Build history of the part. All positions in model axes, mm. A direction names the side the tool comes from. Coordinates: 2 decimals unless noted, no trailing zeros. Loops run counter-clockwise (first coordinate to the right, second up) from the corner with the lowest first, then second, coordinate; pieces in that order, holes last.
(1) Slice it at A-A (y = 4.5). Give the cut face in (x, z), and give its area (3 significant figures).
(2) Two-plate mould, pull along X, no slides. Class faces 1 (the face through (0, -11, 7)), 2 (the face through (-13.887, -10.648, 13.395)): pulls with the +X half, pulls with the -X half, needs draft (parallel to the pull), parting line crosses it, or undercut.
(3) Slice it at D-D (x = -7). Give the cut face in (y, z), and give its area (3 significant figures).
(4) Slice it at B-B (x = 24.5). Give the cut face in (y, z), and give its area (3 significant figures).
(5) Tool access for faces 3 (the face through (9.54, -7.32, 3.45)), 4 (the face through (-29.97, 1.32, 2.46)), 5 (the face through (7.94, 13.6, 16.07)): list every direction of +Z, -Z, +X, -X, +Y, -Y with a clear straight run to the whole face (end or side of a thin tool).
(6) Flat gauge pins, fed straight in: P1, Ø6, axis at x = -3, z = 11, coming from the -Y side; P2, Ø2, axis at x = -4.5, z = 9.5, coming from the +Y side; P3, Ø4, axis at y = -0.5, z = 10.5, coming from the +X side. Where does each tip first touch, or does it go through?
(7) Wall check: L1, parallel to Y at x = 12.25, z = 1.6; L2, parallel to X at y = -13.5, z = 11.75; L3, parallel to Y at x = -11, z = 2.25. Give the ranges that are in metal, low to high.
(8) Slice it at C-C (z = 8.25). Give the cut face in (x, y), and give its area (3 significant figures).
from build123d import *

# Parameters (mm, degrees)
SKETCH1_R           = 30
BOSS_EXTRUDE1_DEPTH = 5
SKETCH2_R           = 19.5
BOSS_EXTRUDE2_DEPTH = 1
SKETCH3_R           = 17.5
BOSS_EXTRUDE3_DEPTH = 15
SKETCH4_R           = 12.025
CUT_EXTRUDE1_DEPTH  = 7
SKETCH5_R           = 10.5
CUT_EXTRUDE2_DEPTH  = 45.676615807
SKETCH6_R           = 1.75
CUT_EXTRUDE3_DEPTH  = 46.343136195
SKETCH7_R           = 1.75
CUT_EXTRUDE4_DEPTH  = 10
SKETCH8_R           = 1.225
CUT_EXTRUDE5_DEPTH  = 12


with BuildPart() as part:
    # Sketch1 → Boss-Extrude1 (new body)
    with BuildSketch(Plane.XY):
        Circle(SKETCH1_R)
    extrude(amount=BOSS_EXTRUDE1_DEPTH)

    # Sketch2 → Boss-Extrude2 (add)
    with BuildSketch(Plane.XY.offset(5)):
        Circle(SKETCH2_R)
    extrude(amount=BOSS_EXTRUDE2_DEPTH)

    # Sketch3 → Boss-Extrude3 (add)
    with BuildSketch(Plane.XY.offset(6)):
        Circle(SKETCH3_R)
    extrude(amount=BOSS_EXTRUDE3_DEPTH)

    # Sketch4 → Cut-Extrude1 (cut)
    with BuildSketch(Plane(origin=(0, 0, 0), x_dir=(-1, 0, 0), z_dir=(0, 0, -1))):
        Circle(SKETCH4_R)
    extrude(amount=-CUT_EXTRUDE1_DEPTH, mode=Mode.SUBTRACT)

    # Sketch5 → Cut-Extrude2 (cut, through all)
    with BuildSketch(Plane(origin=(0, 0, 7), x_dir=(-1, 0, 0), z_dir=(0, 0, -1))):
        Circle(SKETCH5_R)
    extrude(amount=-CUT_EXTRUDE2_DEPTH, mode=Mode.SUBTRACT)

    # Sketch6 → Cut-Extrude3 (cut, through all)
    with BuildSketch(Plane.XY.offset(5)):
        with Locations((24.5, 0)):
            Circle(SKETCH6_R)
        with Locations((12.25, -21.217622393)):
            Circle(SKETCH6_R)
        with Locations((-12.25, -21.217622393)):
            Circle(SKETCH6_R)
        with Locations((-24.5, 0)):
            Circle(SKETCH6_R)
        with Locations((-12.25, 21.217622393)):
            Circle(SKETCH6_R)
        with Locations((12.25, 21.217622393)):
            Circle(SKETCH6_R)
    extrude(amount=-CUT_EXTRUDE3_DEPTH, mode=Mode.SUBTRACT)

    # Sketch7 → Cut-Extrude4 (cut)
    with BuildSketch(Plane.XY.offset(21)):
        with Locations((14, 0)):
            Circle(SKETCH7_R)
        with Locations((7, -12.124355653)):
            Circle(SKETCH7_R)
        with Locations((-7, -12.124355653)):
            Circle(SKETCH7_R)
        with Locations((-14, 0)):
            Circle(SKETCH7_R)
        with Locations((-7, 12.124355653)):
            Circle(SKETCH7_R)
        with Locations((7, 12.124355653)):
            Circle(SKETCH7_R)
    extrude(amount=-CUT_EXTRUDE4_DEPTH, mode=Mode.SUBTRACT)

    # Sketch8 → Cut-Extrude5 (cut)
    with BuildSketch(Plane.XY.offset(21)):
        with Locations((12.124355653, 7)):
            Circle(SKETCH8_R)
        with Locations((0, -14)):
            Circle(SKETCH8_R)
        with Locations((-12.124355653, 7)):
            Circle(SKETCH8_R)
    extrude(amount=-CUT_EXTRUDE5_DEPTH, mode=Mode.SUBTRACT)


solid = part.part
Response values:
1. outline: (-29.66, 0) - (-11.15, 0) - (-11.15, 7) - (-9.49, 7) - (-9.49, 21) - (-16.91, 21) - (-16.91, 6) - (-18.97, 6) - (-18.97, 5) - (-29.66, 5) - close; (9.49, 7) - (11.15, 7) - (11.15, 0) - (29.66, 0) - (29.66, 5) - (18.97, 5) - (18.97, 6) - (16.91, 6) - (16.91, 21) - (9.49, 21) - close
1. area: 420 mm2
2. face 1: undercut
2. face 2: parting line crosses it
3. outline: (-29.17, 0) - (-9.78, 0) - (-9.78, 7) - (-7.83, 7) - (-7.83, 21) - (-10.37, 21) - (-10.37, 11) - (-13.87, 11) - (-13.87, 21) - (-16.04, 21) - (-16.04, 6) - (-18.2, 6) - (-18.2, 5) - (-29.17, 5) - close; (7.83, 7) - (9.78, 7) - (9.78, 0) - (29.17, 0) - (29.17, 5) - (18.2, 5) - (18.2, 6) - (16.04, 6) - (16.04, 21) - (13.87, 21) - (13.87, 11) - (10.37, 11) - (10.37, 21) - (7.83, 21) - close
3. area: 383 mm2
4. outline: (-17.31, 0) - (-1.75, 0) - (-1.75, 5) - (-17.31, 5) - close; (1.75, 0) - (17.31, 0) - (17.31, 5) - (1.75, 5) - close
4. area: 156 mm2
5. face 3: -Z
5. face 4: +Z, -Z
5. face 5: +Z
6. P1: stops at y = -17.5
6. P2: stops at y = 17.15
6. P3: stops at x = 17.5
7. L1: y = -27.38 to -22.97, -19.47 to 19.47, 22.97 to 27.38
7. L2: x = -11.14 to -8.08, -5.92 to -1.12, 1.12 to 5.92, 8.08 to 11.14
7. L3: y = -27.91 to -22.44, -19.99 to -4.86, 4.86 to 19.99, 22.44 to 27.91
8. outline: circle Ø35 at (0, 0); hole circle Ø21 at (0, 0)
8. area: 616 mm2
